```python
from build123d import *

# Parameters (mm, degrees)
SKETCH1_W           = 336
SKETCH1_H           = 115
BOSS_EXTRUDE1_DEPTH = 6.35
CUT_EXTRUDE1_DEPTH  = 6.35


with BuildPart() as part:
    # Sketch1 → Boss-Extrude1 (new body)
    with BuildSketch(Plane.XY):
        with BuildLine():
            Line((145.931677019, 105.5), (-145.931677019, 105.5))
            ThreePointArc((-145.931677019, 105.5), (-162.655478234, 99.082639019), (-170.793465899, 83.125157832))
            Line((-170.793465899, 83.125157832), (-205.004646024, -240.874842168))
            ThreePointArc((-205.004646024, -240.874842168), (-198.725496162, -260.223801216), (-180.142857143, -268.5))
            Line((-180.142857143, -268.5), (180.142857143, -268.5))
            ThreePointArc((180.142857143, -268.5), (198.725496162, -260.223801216), (205.004646024, -240.874842168))
            Line((205.004646024, -240.874842168), (170.793465899, 83.125157832))
            ThreePointArc((170.793465899, 83.125157832), (162.655478234, 99.082639019), (145.931677019, 105.5))
        make_face()
        Polygon((-83, 80.5), (83, 80.5), (107, -80.5), (-100, -80.5), align=None, mode=Mode.SUBTRACT)
        with Locations((0, -186)):
            Rectangle(SKETCH1_W, SKETCH1_H, mode=Mode.SUBTRACT)
    extrude(amount=BOSS_EXTRUDE1_DEPTH)

    # Sketch2 → Cut-Extrude1 (cut)
    with BuildSketch(Plane.XY.offset(6.35)):
        Polygon((-102.222298481, -82.5), (109.320235916, -82.5), (84.723962625, 82.5), (-84.799938233, 82.5), align=None)
    extrude(amount=-CUT_EXTRUDE1_DEPTH, mode=Mode.SUBTRACT)


solid = part.part
```
Geometry: final body of the model. Coordinates: model frame, mm. A direction names the side the tool comes from. Give positions to 0.01 mm unless a question says otherwise; leave off trailing zeros. Order: outer loops, then holes, each group sorted by start corner. A loop starts at its lowest first (then second) coordinate and runs counter-clockwise, first axis right, second up. Notation, with made-up numbers: (-20, 85) -> (33, 85) arc R25 cw to (33, 116) -> close; hole circle Ø2 at (73, -35). An arc over 180 degrees is marked (long way). Write each question's results on one line, items separated by ' | '. Start each with the question number.
1) First-contact query: pin 1 (1.5 mm diameter, centred on y = -27.5, z = 3.5, fed in from -X). Flat tip, straight axial feed; report the tip coordinate or a pass-through.
2) Section C-C (y = -164.5). Return loops of the section in (x, z), then the cut area to 3 significant figures.
3) Draft query along Y for faces 3 (the flat face through (-3, -120, 6.35)), 4 (the cylindrical face through (-162.464, 99.253, 3.131)), 5 (the flat face through (-93.39, 1.15, 3.22)). Return one class per face: pulls with the +Y half, pulls with the -Y half, needs draft (parallel to the pull), parting line crosses it, or undercut.
4) Set-up query: faces 1 (the flat face through (-187.66, -76.61, 3.13)), 2 (the flat face through (97.2, -1.2, 3.2)). Return all of +Z, -Z, +X, -X, +Y, -Y with unobstructed straight access to the full face (end or side cutting, diameter ignored); none if empty.
5) Section A-A (x = -114). Return loops of the section in (y, z), then the cut area to 3 significant figures.
6) Section B-B (z = 5). Return loops of the section in (x, y), then the cut area to 3 significant figures.
7) Line query: line 1 (Y direction, x = 84.5, z = 2); line 2 (Y direction, x = -123, z = 3.75); line 3 (X direction, y = -9.5, z = 2.5). Output: solid intervals per line, ascending. Write a range as from..to.
Calculated:
1) pin 1: x = -182.55
2) outline: (-196.94, 0) -> (-168, 0) -> (-168, 6.35) -> (-196.94, 6.35) -> close; (168, 0) -> (196.94, 0) -> (196.94, 6.35) -> (168, 6.35) -> close | area: 368 mm2
3) face 3: needs draft | face 4: pulls with the +Y half | face 5: undercut
4) face 1: +Z, -Z, -X, +Y | face 2: +Z, -Z
5) outline: (-268.5, 0) -> (-243.5, 0) -> (-243.5, 6.35) -> (-268.5, 6.35) -> close; (-128.5, 0) -> (105.5, 0) -> (105.5, 6.35) -> (-128.5, 6.35) -> close | area: 1,640 mm2
6) outline: (-205, -240.87) arc R25 ccw to (-180.14, -268.5) -> (180.14, -268.5) arc R25 ccw to (205, -240.87) -> (170.79, 83.13) arc R25 ccw to (145.93, 105.5) -> (-145.93, 105.5) arc R25 ccw to (-170.79, 83.13) -> close; hole (-168, -243.5) -> (168, -243.5) -> (168, -128.5) -> (-168, -128.5) -> close; hole (-102.22, -82.5) -> (109.32, -82.5) -> (84.72, 82.5) -> (-84.8, 82.5) -> close | area: 70,100 mm2
7) line 1: -268.5..-243.5, -128.5..-82.5, 82.5..105.5 | line 2: -268.5..-243.5, -128.5..105.5 | line 3: -180.57..-94.51, 98.44..180.57
